Geometry check sheet. Reference: the model listing, model coordinates, mm. Face numbers are marked on the shaded views. Coordinates: 2 decimals unless noted, no trailing zeros. Write each loop counter-clockwise with the first axis right and the second up, starting at its lowest first coordinate (ties: lowest second). Pieces come first, ordered by that corner, then holes. Notation, with made-up numbers: (71.25, -20) -> (100.25, -20) arc R26 ccw to (100.25, 13) -> close; hole circle Ø3 at (10.5, 84.5). An arc over 180 degrees is marked (long way). One line per question, with ' | ' between items.
```python
from build123d import *

# Parameters (mm, degrees)
SKETCH1_R           = 1.5
BOSS_EXTRUDE1_DEPTH = 3.48
SHELL1_T            = -2


with BuildPart() as part:
    # Sketch1 → Boss-Extrude1 (new body)
    with BuildSketch(Plane(origin=(0, 0, 0), x_dir=(1, 0, 0), z_dir=(0, 1, 0))):
        Polygon((84.974878237, 39.0892), (64.974878237, 39.0892), (39.398878237, 22.738080915), (39.398878237, -22.738080915), (64.974878237, -39.0892), (84.974878237, -39.0892), align=None)
        with Locations((45.898878237, 19.1788)):
            Circle(SKETCH1_R, mode=Mode.SUBTRACT)
        with Locations(Location((45.898878237, -19.1788, 0), (0, 0, 90))):
            Circle(SKETCH1_R, mode=Mode.SUBTRACT)
    extrude(amount=BOSS_EXTRUDE1_DEPTH)

    # Shell1
    shell1_openings = [part.faces().sort_by_distance(p)[0] for p in [
        (64.165608006, 3.48, 0),
    ]]
    offset(amount=SHELL1_T, openings=shell1_openings, kind=Kind.INTERSECTION)


solid = part.part
```
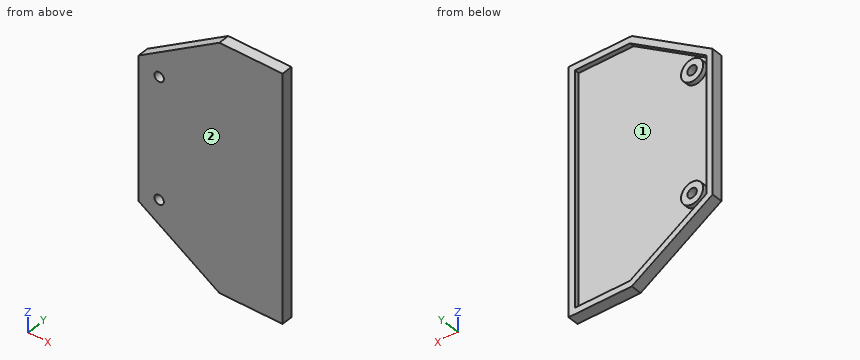
(1) Draft check along X on the marked faces 1 and 2. Enter one of: pulls with the +X half, pulls with the -X half, needs draft (parallel to the pull), parting line crosses it, or undercut.
Answers below:
face 1: undercut | face 2: needs draft
(2) Material ranges on line 1 (X direction, y = 2.9, z = 0); line 2 (Z direction, x = 77, y = 2.95); line 3 (Z direction, x = 46, y = 2.4), recorded low to high.
Answers below:
line 1: x = 39.4 to 41.4, 82.97 to 84.97 | line 2: z = -39.09 to -37.09, 37.09 to 39.09 | line 3: z = -26.96 to -24.58, -22.68 to -20.68, -17.68 to -15.68, 15.68 to 17.68, 20.68 to 22.68, 24.58 to 26.96
(3) Cross-section at D-D (x = 43.5). Record the cut outline in (y, z), plus the area to 3 significant figures.
Answers below:
outline: (0, -25.36) -> (3.48, -25.36) -> (3.48, -22.99) -> (2, -22.99) -> (2, -21.73) -> (3.48, -21.73) -> (3.48, -16.63) -> (2, -16.63) -> (2, 16.63) -> (3.48, 16.63) -> (3.48, 21.73) -> (2, 21.73) -> (2, 22.99) -> (3.48, 22.99) -> (3.48, 25.36) -> (0, 25.36) -> close | area: 124 mm²
(4) Depth check by flat-ended pin: P1, Ø1.5, axis at x = 55.5, z = -25, coming from the +Y side. Enter the tip coordinate at first touch or a pass-through.
Answers below:
P1: stops at y = 2
(5) Cross-section at A-A (z = 10). Record the cut outline in (x, y), plus the area to 3 significant figures.
Answers below:
outline: (39.4, 0) -> (84.97, 0) -> (84.97, 3.48) -> (82.97, 3.48) -> (82.97, 2) -> (41.4, 2) -> (41.4, 3.48) -> (39.4, 3.48) -> close | area: 97.1 mm²
(6) Cross-section at C-C (x = 81.5). Record the cut outline in (y, z), plus the area to 3 significant figures.
Answers below:
outline: (0, -39.09) -> (3.48, -39.09) -> (3.48, -37.09) -> (2, -37.09) -> (2, 37.09) -> (3.48, 37.09) -> (3.48, 39.09) -> (0, 39.09) -> close | area: 162 mm²
(7) Cross-section at B-B (y = 1.15). Record the cut outline in (x, z), plus the area to 3 significant figures.
Answers below:
outline: (39.4, -22.74) -> (64.97, -39.09) -> (84.97, -39.09) -> (84.97, 39.09) -> (64.97, 39.09) -> (39.4, 22.74) -> close; hole circle Ø3 at (45.9, -19.18); hole circle Ø3 at (45.9, 19.18) | area: 3,130 mm²
